The model under review builds one solid part; all positions refer to its coordinate system, in mm. Face numbers are marked on the shaded views. A direction names the side the tool comes from. Give positions to 0.01 mm unless a question says otherwise; leave off trailing zeros. Order: outer loops, then holes, each group sorted by start corner. A loop starts at its lowest first (then second) coordinate and runs counter-clockwise, first axis right, second up.
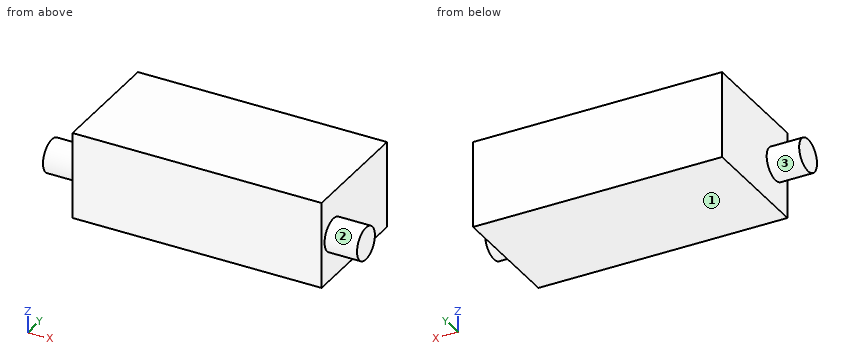
```python
from build123d import *

# Parameters (mm, degrees)
SKETCH1_W           = 146.05
SKETCH1_H           = 50.8
BOSS_EXTRUDE1_DEPTH = 69.85
SKETCH2_R           = 9.525
BOSS_EXTRUDE2_DEPTH = 19.05
BOSS_EXTRUDE3_START = 19.05
SKETCH3_R           = 9.525
BOSS_EXTRUDE3_DEPTH = 19.05


with BuildPart() as part:
    # Sketch1 → Boss-Extrude1 (new body)
    with BuildSketch(Plane(origin=(0, 0, 0), x_dir=(1, 0, 0), z_dir=(0, 1, 0))):
        with Locations((73.025, 25.4)):
            Rectangle(SKETCH1_W, SKETCH1_H)
    extrude(amount=BOSS_EXTRUDE1_DEPTH)

    # Sketch2 → Boss-Extrude2 (add)
    with BuildSketch(Plane(origin=(146.05, 0, 0), x_dir=(0, 0, -1), z_dir=(1, 0, 0))):
        with Locations(Location((25.4, 12.7, 0), (0, 0, 180))):
            Circle(SKETCH2_R)
    extrude(amount=BOSS_EXTRUDE2_DEPTH)

    # Sketch3 → Boss-Extrude3 (add)
    with BuildSketch(Plane.ZY.offset(BOSS_EXTRUDE3_START)):
        with Locations((-25.4, 12.7)):
            Circle(SKETCH3_R)
    extrude(amount=-BOSS_EXTRUDE3_DEPTH)


solid = part.part
```
1. Take a section at A-A (z = -25.4). Write out the cut boundary in (x, y) (3 decimals), and give its area (3 significant figures).
2. To check wall thickness, follow line 1 (X direction, y = 44, z = -48); line 2 (Z direction, x = -8, y = 12.5); line 3 (Z direction, x = -5.5, y = 21). State the ranges of each line that lie inside material, in increasing order.
3. For the marked faces 1, 2 and 3, list the 3-axis set-ups (+Z, -Z, +X, -X, +Y, -Y) from which the entire face can be reached by the end or side of a thin tool; tool diameter is ignored.
4. Take a section at C-C (x = -5.5). Write out the cut boundary in (y, z) (3 decimals).
5. Insertion check: pin 1 (5 mm diameter, centred on y = 56, z = -12, fed in from +X); pin 2 (6 mm diameter, centred on y = 41, z = -41.5, fed in from -X). Each pin has a flat end and moves straight along its axis. Give the tip position at first contact, or say it passes through.
6. Take a section at D-D (z = -41). Write out the cut boundary in (x, y), and give its area (3 significant figures).
7. Take a section at B-B (y = 12.7). Write out the cut boundary in (x, z) (3 decimals).
Answer:
1. outline: (-19.05, 3.175) - (0, 3.175) - (0, 0) - (146.05, 0) - (146.05, 3.175) - (165.1, 3.175) - (165.1, 22.225) - (146.05, 22.225) - (146.05, 69.85) - (0, 69.85) - (0, 22.225) - (-19.05, 22.225) - close
1. area: 10,900 mm2
2. line 1: x = 0 to 146.05
2. line 2: z = -34.92 to -15.88
2. line 3: z = -30.07 to -20.73
3. face 1: -Z, +X, -X, +Y, -Y
3. face 2: +X
3. face 3: -X
4. outline: circle Ø19.05 at (12.7, -25.4)
5. pin 1: stops at x = 146.05
5. pin 2: stops at x = 0
6. outline: (0, 0) - (146.05, 0) - (146.05, 69.85) - (0, 69.85) - close
6. area: 10,200 mm2
7. outline: (-19.05, -34.925) - (0, -34.925) - (0, -50.8) - (146.05, -50.8) - (146.05, -34.925) - (165.1, -34.925) - (165.1, -15.875) - (146.05, -15.875) - (146.05, 0) - (0, 0) - (0, -15.875) - (-19.05, -15.875) - close
